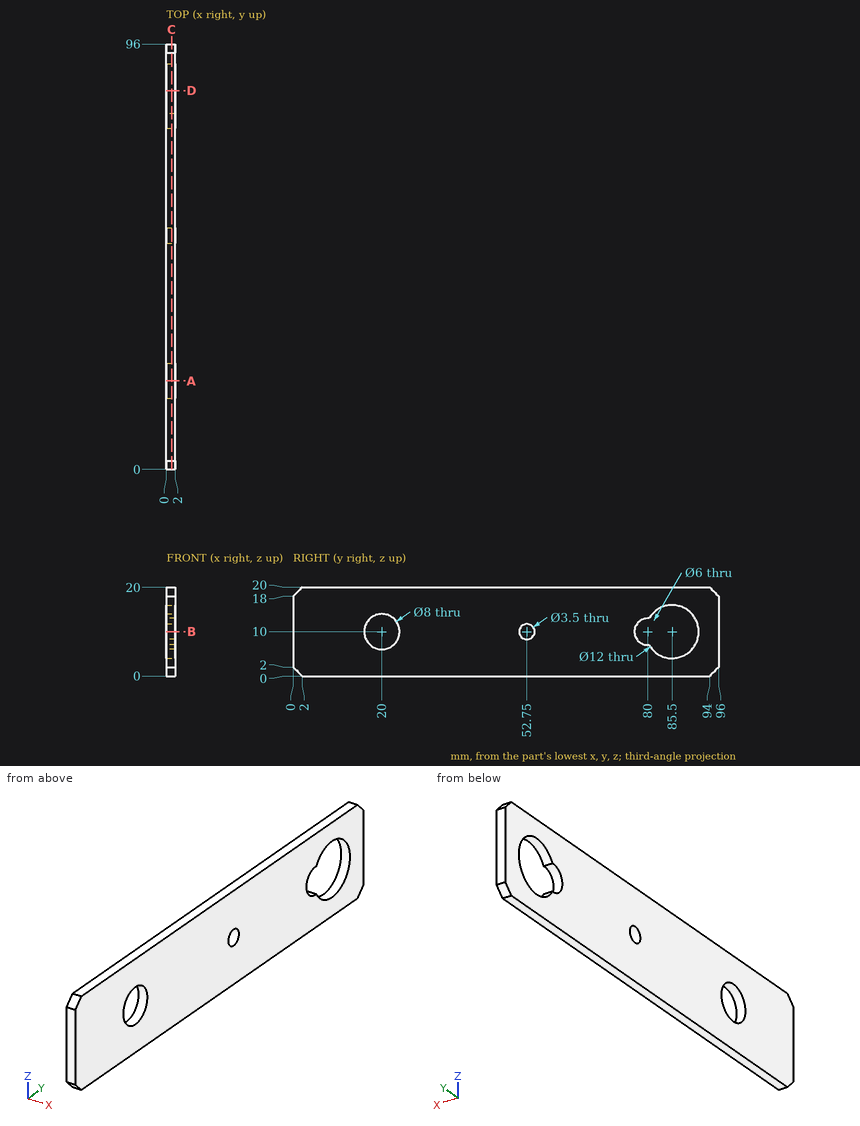
Geometry: see drawing. Coordinates: mm, zero at the bounding-box minimum. Round coordinates to 2 decimals unless told otherwise and drop trailing zeros. Loops run counter-clockwise (first coordinate to the right, second up) from the corner with the lowest first, then second, coordinate; pieces in that order, holes last. Notation, with made-up numbers: (-22, 25) -> (12, 25) arc R17 cw to (12, 43) -> close; hole circle Ø1 at (38.25, 69.25). An arc over 180 degrees is marked (long way). One line per question, with ' | ' between items. Start each with the question number.
1. Line query: line 1 along Z through (x, y) = (0.65, 80); line 2 along Y through (x, z) = (0.7, 12.25); line 3 along Z through (x, y) = (0.45, 85.5). Output: solid intervals per line, ascending. Write a range as [from, to].
2. Section B-B on z = 10. Output: boundary loops of the cut face in (x, y), and give its area (3 significant figures).
3. Section C-C on x = 1.2. Output: boundary loops of the cut face in (y, z).
4. Section D-D on y = 85.5. Output: boundary loops of the cut face in (x, z).
5. Section A-A on y = 20. Output: boundary loops of the cut face in (x, z), and give its area (3 significant figures).
Returned:
1) line 1: z = [0, 7], [13, 20] | line 2: y = [0, 16.69], [23.31, 78.02], [91.06, 96] | line 3: z = [0, 4], [16, 20]
2) outline: (0, 0) -> (2, 0) -> (2, 16) -> (0, 16) -> close; (0, 24) -> (2, 24) -> (2, 51) -> (0, 51) -> close; (0, 54.5) -> (2, 54.5) -> (2, 77) -> (0, 77) -> close; (0, 91.5) -> (2, 91.5) -> (2, 96) -> (0, 96) -> close | area: 140 mm2
3) outline: (0, 2) -> (2, 0) -> (94, 0) -> (96, 2) -> (96, 18) -> (94, 20) -> (2, 20) -> (0, 18) -> close; hole circle Ø8 at (20, 10); hole circle Ø3.5 at (52.75, 10); hole (80.3, 7.01) arc R6 ccw (long way) to (80.3, 12.99) arc R3 ccw (long way) to start
4) outline: (0, 0) -> (2, 0) -> (2, 4) -> (0, 4) -> close; (0, 16) -> (2, 16) -> (2, 20) -> (0, 20) -> close
5) outline: (0, 0) -> (2, 0) -> (2, 6) -> (0, 6) -> close; (0, 14) -> (2, 14) -> (2, 20) -> (0, 20) -> close | area: 24.0 mm2
